Solid Edge part; units mm, degrees
sketch "Sketch1" plane through (0, 0, 0) normal (0, 0, 1) x (1, 0, 0)
  line L0 (-60, 0) -> (30, -51.9615)
  line L1 (30, -51.9615) -> (30, 51.9615)
  line L2 (30, 51.9615) -> (-60, 0)
extrude "Protrusion1" add sketch "Sketch1" along normal up to vertex (84.8528 mm away)
sketch "Sketch2" plane through (0, 0, 0) normal (0, -1, 0) x (1, 0, 0)
  line L0 (0, 84.8528) -> (30, 0)
extrude "Cutout1" cut sketch "Sketch2" along normal mid plane 103.923 material side at (15.0471, 0, 42.4431)
pattern_circular "Pattern1" count 3 over 360 about axis through (0, 0, 0) along (0, 0, -1) of "Cutout1"
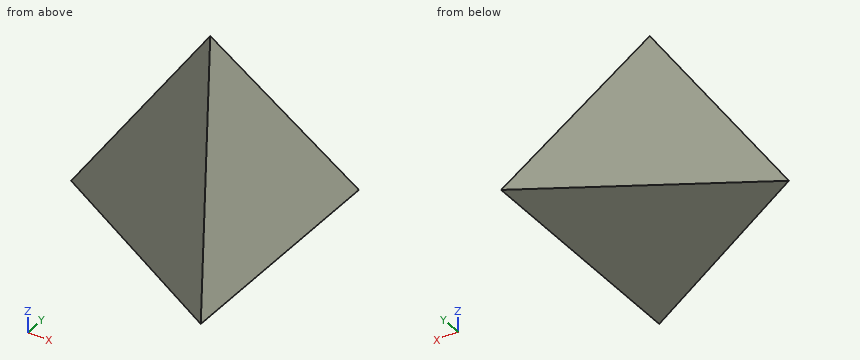
Work out the finished part from the listing and answer in its coordinate system (mm). Coordinates: 2 decimals unless noted, no trailing zeros. Write each loop counter-clockwise with the first axis right and the second up, starting at its lowest first coordinate (ties: lowest second). Pieces come first, ordered by that corner, then holes.
Q1. A cutting plane is placed at C-C, the plane x = 7. Give the vertices of the cut face in (y, z), then the cut area to 3 significant figures.
Q2. A cutting plane is placed at B-B, the plane z = 12.5. Give the vertices of the cut face in (x, y), then the cut area to 3 significant figures.
Q3. Each of these flat-tipped pins is pushed along its axis until it touches: pin 1 Ø3 at (x, z) = (-13, 35.5) entering from +Y; pin 2 Ø12 at (y, z) = (6, 38) entering from +X; pin 3 Ø5 at (x, z) = (-17, 50.5) entering from -Y. Where does it stop, or does it pass through?
Q4. A cutting plane is placed at D-D, the plane x = 17. Give the vertices of the cut face in (y, z), then the cut area to 3 significant figures.
Q5. A cutting plane is placed at A-A, the plane y = 21.5. Give the vertices of the cut face in (x, z).
Q6. Find the intervals of material crossed by line 1 (Y direction, x = 6.5, z = 48); line 2 (Y direction, x = -10, z = 39); line 3 (X direction, y = 1, z = 79), in increasing order.
Findings below:
1. outline: (-38.68, 0) - (38.68, 0) - (12.12, 65.05) - (-12.12, 65.05) - close
1. area: 3,310 mm2
2. outline: (-51.16, 0) - (25.58, -44.31) - (25.58, 44.31) - close
2. area: 3,400 mm2
3. pin 1: stops at y = 13.7
3. pin 2: stops at x = 18.69
3. pin 3: stops at y = -5.98
4. outline: (-44.46, 0) - (44.46, 0) - (29.44, 36.77) - (-29.44, 36.77) - close
4. area: 2,720 mm2
5. outline: (-22.76, 0) - (30, 0) - (12.41, 49.74) - close
6. line 1: y = -18.8 to 18.8
6. line 2: y = -12.95 to 12.95
6. line 3: x = -2.41 to 2.07
